from build123d import *

# Parameters (mm, degrees)
F0_R     = 9.1524845949
F1_DEPTH = 20
F2_R     = 3.008201979
F3_DEPTH = 110
F4_R     = 9.1770067028
F5_DEPTH = 20
F7_R     = 2.5


# Not quite as in the source:
# - a fillet or chamfer that OpenCascade refuses, or shapes differently, is made with other operations: its cross-section is extruded or revolved along the edge and cut away or added


with BuildPart() as f1:
    # F0 (on Top) → F1 (new body)
    with BuildSketch(Plane.XY):
        Circle(F0_R)
    extrude(amount=F1_DEPTH)

    # F2 (on face) → F3 (join)
    with BuildSketch(Plane.XY.offset(20)):
        Circle(F2_R)
    extrude(amount=F3_DEPTH)

    # F4 (on face) → F5 (join)
    with BuildSketch(Plane.XY.offset(130)):
        Circle(F4_R)
    extrude(amount=F5_DEPTH)

    # F6: fillet of radius 7.5 on 2 edges, made by hand

    # F6_s1 → F6_t2 (revolve, cut)
    with BuildSketch(Plane.XZ):
        with BuildLine():
            ThreePointArc((3.008201979, 20), (7.4152044554, 17.4236593265), (9.1524845949, 12.6235489309))
            Line((9.1524845949, 12.6235489309), (9.1524845949, 20))
            Line((9.1524845949, 20), (3.008201979, 20))
        make_face()
    revolve(axis=Axis((0, 0, 20), (0, 0, 1)), mode=Mode.SUBTRACT)

    # F6_s3 → F6_t4 (revolve, cut)
    with BuildSketch(Plane.XZ):
        with BuildLine():
            ThreePointArc((9.1770067028, 137.3809158738), (7.4317423427, 132.5712362884), (3.008201979, 130))
            Line((3.008201979, 130), (9.1770067028, 130))
            Line((9.1770067028, 130), (9.1770067028, 137.3809158738))
        make_face()
    revolve(axis=Axis((0, 0, 130), (0, 0, 1)), mode=Mode.SUBTRACT)

    # F7
    f7_edges = [f1.edges().sort_by_distance(p)[0] for p in [
        (-9.177007, 0, 150),
        (-9.152485, 0, 0),
    ]]
    fillet(f7_edges, radius=F7_R)


solid = f1.part
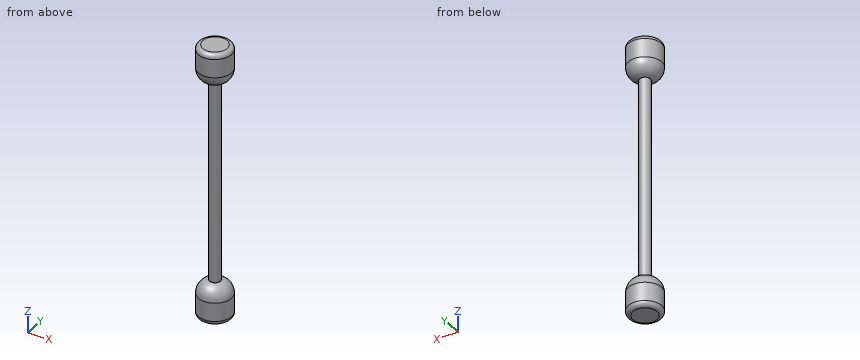
Model file for the job. Use its own axes, mm. Round coordinates to 2 decimals unless told otherwise and drop trailing zeros. Order: outer loops, then holes, each group sorted by start corner. A loop starts at its lowest first (then second) coordinate and runs counter-clockwise, first axis right, second up. Notation, with made-up numbers: M 5,86.5 L 52,86.5 A23 cw 52,94.5 Z; hole C 40.25,-31 d7. An arc over 180 degrees is marked long. Write each question's results on one line, items separated by ' | '. Start each with the question number.
(1) Probe probe 1 along Z at (x, y) = (6, -5.25); probe 2 along Z at (x, y) = (2.5, 5.5); probe 3 along Y at (x, z) = (0, 136.5). List the from-to ranges inside material, lowest first. Write a range as from..to.
(2) Saw through at A-A, the plane z = 49. Give the cut face in (x, y), then the cut area to 3 significant figures.
(3) Drop flat-ended pins along their axis: pin 1 (5 mm diameter, centred on x = -2.5, z = 119.5, fed in from +Y); pin 2 (5 mm diameter, centred on x = -2, z = 107.5, fed in from -Y); pin 3 (4 mm diameter, centred on y = -4.5, z = 134.5, fed in from +X). Give the stop position or say it passes through.
Established:
1) probe 1: z = 0.38..16.66, 133.3..149.64 | probe 2: z = 0..18.71, 131.28..150 | probe 3: y = -9.13..9.13
2) outline: C 0,0 d6.02 | area: 28.4 mm^2
3) pin 1: stops at y = 3.01 | pin 2: stops at y = -3.01 | pin 3: stops at x = 8.51
